Build history of the part. All positions in model axes, mm. A direction names the side the tool comes from. Give positions to 0.01 mm unless a question says otherwise; leave off trailing zeros. Order: outer loops, then holes, each group sorted by start corner. A loop starts at its lowest first (then second) coordinate and runs counter-clockwise, first axis right, second up. Notation, with made-up numbers: (14.25, -6) -> (57.25, -6) arc R15 ccw to (57.25, 19) -> close; hole circle Ø10 at (27, 32). An arc over 180 degrees is marked (long way). One line per question, with ' | ' between items. Start each with the question number.
(1) Which spindle directions (+Z, -Z, +X, -X, +Y, -Y) get a long thin tool onto all of the face, cutting with end or side? Do faces 1 (the face through (10, -30, 23)), 2 (the face through (-23, -33, 41)), 3 (the face through (-14, -35, 50)), 4 (the face through (-25.1, -30.14, 22.86)), 5 (the face through (25.86, -30.14, 26.1)). Say none if no direction does.
(2) Cut at A-A (z = 66). Give the cut face in (x, y).
(3) Pin check, flat tips, straight feed: pin 1 Ø1.5 at (y, z) = (-38, 41.5) entering from -X; pin 2 Ø24 at (x, z) = (-41, 51.5) entering from -Y; pin 3 Ø2.5 at (x, z) = (-23, 74) entering from +Y; pin 4 Ø10.5 at (x, y) = (-37, -24) entering from -Z. Stop position of each tip, or through.
(4) Pull direction Y, two halves, no side cores. Call faces 6 (the face through (15, -30, 77)), 7 (the face through (-21, -34, 50)), 8 (the face through (15, -40, 74)): +Y half, -Y half, draft (parallel to the pull), parting line (faces both ways), or undercut.
(5) Cut at D-D (x = -48.5). Give the cut face in (y, z).
(6) Drill centre lines: L1, parallel to X at y = -26.5, z = 74; L2, parallel to X at y = -30.25, z = 28; L3, parallel to Y at x = -18, z = 64.5. Where is each one in solid material? Low to high. Write a range as from..to.
(7) Cut at B-B (y = -38). Give the cut face in (x, z).
(8) Cut at C-C (y = -26.5). Give the number of separate pieces and of enclosed holes in the cut face, then the cut area to 3 significant figures.
from build123d import *

# Parameters (mm, degrees)
EXTRUDE_1_DEPTH             = 10
EXTRUDE_2_REACH             = 34.619
SKETCH_2_R                  = 10
EXTRUDE_2_DIRECTION_2_DEPTH = 2
SKETCH_6_R                  = 1.65
SKETCH_6_W                  = 14.704506527
SKETCH_6_H                  = 8.520368268
CUT_EXTRUDE_2_DEPTH         = 43.983979574
FILLET_1_R                  = 1
FILLET_2_R                  = 0.5
EXTRUDE_3_DEPTH             = 8
EXTRUDE_4_DEPTH             = 55
SKETCH_9_W                  = 73
SKETCH_9_H                  = 45
CUT_EXTRUDE_3_DEPTH         = 13
SKETCH_10_W                 = 15
SKETCH_10_H                 = 20
CUT_EXTRUDE_4_DEPTH         = 13
SKETCH_11_W                 = 73
SKETCH_11_H                 = 45
CUT_EXTRUDE_6_DEPTH         = 13
SKETCH_12_W                 = 15
SKETCH_12_H                 = 45
SKETCH_12_W_2               = 10
EXTRUDE_5_DEPTH             = 5
FILLET_3_R                  = 3
SKETCH_14_R                 = 1.55
CUT_EXTRUDE_7_DEPTH         = 102.004950374
SKETCH_15_W                 = 8
SKETCH_15_H                 = 22
CUT_EXTRUDE_8_DEPTH         = 20
SKETCH_18_W                 = 5
SKETCH_18_H                 = 45
SKETCH_18_W_2               = 30.3
EXTRUDE_6_DEPTH             = 13
SKETCH_20_R                 = 1.5
CUT_EXTRUDE_9_DEPTH         = 13


with BuildPart() as part:
    # 草图1 → 凸台-拉伸1 (new, symmetric)
    with BuildSketch(Plane.XY):
        with BuildLine():
            Line((-1.15, 3.987480407), (-1.15, 12))
            Line((-1.15, 12), (-4.15, 12))
            Line((-4.15, 12), (-4.15, 4.333301282))
            ThreePointArc((-4.15, 4.333301282), (-4.784308974, 3.620826928), (-5.297685557, 2.816829377))
            Line((-5.297685557, 2.816829377), (-8, -2.265484914))
            Line((-8, -2.265484914), (-8, -30))
            Line((-8, -30), (0, -30))
            Line((0, -30), (0, -8.485281374))
            Line((0, -8.485281374), (4.242640687, -4.242640687))
            ThreePointArc((4.242640687, -4.242640687), (5.999649956, 0.064810571), (4.15, 4.333301282))
            Line((4.15, 4.333301282), (4.15, 12))
            Line((4.15, 12), (1.15, 12))
            Line((1.15, 12), (1.15, 3.987480407))
            ThreePointArc((1.15, 3.987480407), (0, -4.15), (-1.15, 3.987480407))
        make_face()
    extrude(amount=EXTRUDE_1_DEPTH, both=True)

    # 凸台-拉伸2: up to this face of the body (flat: up to its plane)
    extrude_2_end = Plane(part.part.faces().sort_by_distance((-8, -16.132742457, 0))[0])
    # 草图2 → 凸台-拉伸2 (add, up to the picked face)
    with BuildSketch(Plane(origin=(0, 0, 0), x_dir=(0, 0, -1), z_dir=(1, 0, 0)), mode=Mode.PRIVATE) as extrude_2_sk1:
        with Locations((0, -30)):
            Circle(SKETCH_2_R)
    extrude_2_tool1 = split(extrude(extrude_2_sk1.sketch, amount=-EXTRUDE_2_REACH, mode=Mode.PRIVATE), bisect_by=extrude_2_end, keep=Keep.BOTH, mode=Mode.PRIVATE)
    add(extrude_2_tool1.solids().sort_by(Axis((0, -30, 0), (-1, 0, 0)))[0])

    # 草图2 → 凸台-拉伸2 direction 2 (add)
    with BuildSketch(Plane(origin=(0, 0, 0), x_dir=(0, 0, -1), z_dir=(1, 0, 0))):
        with Locations((0, -30)):
            Circle(SKETCH_2_R)
    extrude(amount=EXTRUDE_2_DIRECTION_2_DEPTH)

    # 草图6 → 切除-拉伸2 (cut, through all)
    with BuildSketch(Plane(origin=(4.15, 0, 0), x_dir=(0, 0, -1), z_dir=(1, 0, 0))):
        with Locations(Location((0, 9.5, 0), (0, 0, 90))):
            Circle(SKETCH_6_R)
        with Locations((-12.852253263, 11.760184134)):
            Rectangle(SKETCH_6_W, SKETCH_6_H)
        with Locations((12.852253263, 11.760184134)):
            Rectangle(SKETCH_6_W, SKETCH_6_H)
    extrude(amount=-CUT_EXTRUDE_2_DEPTH, mode=Mode.SUBTRACT)

    # 圆角1
    fillet_1_edges = [part.edges().sort_by_distance(p)[0] for p in [
        (2.65, 7.5, -10),
        (-2.65, 7.5, -10),
        (2.65, 7.5, 10),
        (-2.65, 7.5, 10),
        (2.65, 12, 5.5),
        (-2.65, 12, 5.5),
        (2.65, 12, -5.5),
        (-2.65, 12, -5.5),
    ]]
    fillet(fillet_1_edges, radius=FILLET_1_R)

    # 圆角2
    fillet_2_edges = [part.edges().sort_by_distance(p)[0] for p in [
        (-2.65, 7.5, 5.5),
        (2.65, 7.5, 5.5),
        (2.65, 7.5, -5.5),
        (-2.65, 7.5, -5.5),
    ]]
    fillet(fillet_2_edges, radius=FILLET_2_R)

    # 草图7 → 凸台-拉伸3 (add)
    with BuildSketch(Plane(origin=(2, 0, 0), x_dir=(0, 0, -1), z_dir=(1, 0, 0))):
        with BuildLine():
            Line((0, -20), (-22, -20))
            Line((-22, -20), (-22, -40))
            Line((-22, -40), (0, -40))
            ThreePointArc((0, -40), (10, -30), (0, -20))
        make_face()
    extrude(amount=EXTRUDE_3_DEPTH)

    # 草图8 → 凸台-拉伸4 (add)
    with BuildSketch(Plane.XY.offset(22)):
        Polygon((10, -20), (-26, -20), (-26, -40), (2, -40), (57, -40), (57, -20), align=None)
    extrude(amount=EXTRUDE_4_DEPTH)

    # 草图9 → 切除-拉伸3 (cut)
    with BuildSketch(Plane(origin=(0, -20, 0), x_dir=(1, 0, 0), z_dir=(0, 1, 0))):
        with Locations((15.5, -49.5)):
            Rectangle(SKETCH_9_W, SKETCH_9_H)
    extrude(amount=-CUT_EXTRUDE_3_DEPTH, mode=Mode.SUBTRACT)

    # 草图10 → 切除-拉伸4 (cut)
    with BuildSketch(Plane(origin=(0, 0, 22), x_dir=(-1, 0, 0), z_dir=(0, 0, -1))):
        with Locations((-17.5, -30)):
            Rectangle(SKETCH_10_W, SKETCH_10_H)
    extrude(amount=-CUT_EXTRUDE_4_DEPTH, mode=Mode.SUBTRACT)

    # 草图11 → 切除-拉伸6 (cut)
    with BuildSketch(Plane(origin=(0, -33, 0), x_dir=(1, 0, 0), z_dir=(0, 1, 0))):
        with Locations((15.5, -49.5)):
            Rectangle(SKETCH_11_W, SKETCH_11_H)
    extrude(amount=-CUT_EXTRUDE_6_DEPTH, mode=Mode.SUBTRACT)

    # 草图12 → 凸台-拉伸5 (add)
    with BuildSketch(Plane.XZ.offset(40)):
        with Locations((-13.5, 49.5)):
            Rectangle(SKETCH_12_W, SKETCH_12_H)
        with Locations((47, 49.5)):
            Rectangle(SKETCH_12_W_2, SKETCH_12_H)
    extrude(amount=-EXTRUDE_5_DEPTH)

    # 圆角3
    fillet_3_edges = [part.edges().sort_by_distance(p)[0] for p in [
        (-26, -30, 22),
        (57, -30, 22),
        (-26, -30, 77),
        (57, -30, 77),
        (10, -30, 27),
        (25, -30, 27),
    ]]
    fillet(fillet_3_edges, radius=FILLET_3_R)

    # 草图14 → 切除-拉伸7 (cut, through all)
    with BuildSketch(Plane(origin=(0, -20, 0), x_dir=(1, 0, 0), z_dir=(0, 1, 0))):
        with Locations(Location((-23, -25, 0), (0, 0, 270))):
            Circle(SKETCH_14_R)
        with Locations(Location((54, -25, 0), (0, 0, 270))):
            Circle(SKETCH_14_R)
        with Locations(Location((-23, -74, 0), (0, 0, 270))):
            Circle(SKETCH_14_R)
        with Locations(Location((54, -74, 0), (0, 0, 270))):
            Circle(SKETCH_14_R)
    extrude(amount=-CUT_EXTRUDE_7_DEPTH, mode=Mode.SUBTRACT)

    # 草图15 → 切除-拉伸8 (cut)
    with BuildSketch(Plane(origin=(0, -20, 0), x_dir=(1, 0, 0), z_dir=(0, 1, 0))):
        with Locations((6, -11)):
            Rectangle(SKETCH_15_W, SKETCH_15_H)
    extrude(amount=-CUT_EXTRUDE_8_DEPTH, mode=Mode.SUBTRACT)


with BuildPart() as body_2:
    # of the pieces the cut leaves, the one that is kept (cut_extrude_8_keep)
    add(part.part.solids().sort_by_distance((-26, -20, 25))[0])

    # 草图18 → 凸台-拉伸6 (add)
    with BuildSketch(Plane(origin=(0, -20, 0), x_dir=(1, 0, 0), z_dir=(0, 1, 0))):
        with Locations((-18.5, -49.5)):
            Rectangle(SKETCH_18_W, SKETCH_18_H)
        with Locations((-41.15, -49.5)):
            Rectangle(SKETCH_18_W_2, SKETCH_18_H)
    extrude(amount=-EXTRUDE_6_DEPTH)

    # 草图20 → 切除-拉伸9 (cut)
    with BuildSketch(Plane(origin=(0, -20, 0), x_dir=(1, 0, 0), z_dir=(0, 1, 0))):
        with Locations(Location((-22.89532608, -62.69503523, 0), (0, 0, 270))):
            Circle(SKETCH_20_R)
        with Locations(Location((-51.895321909, -41.179481559, 0), (0, 0, 270))):
            Circle(SKETCH_20_R)
        with Locations((-21.949220364, 0)):
            Circle(SKETCH_20_R)
        with Locations(Location((-51.895321909, -62.69503523, 0), (0, 0, 270))):
            Circle(SKETCH_20_R)
        with Locations(Location((-22.89532608, -41.19503523, 0), (0, 0, 270))):
            Circle(SKETCH_20_R)
    extrude(amount=-CUT_EXTRUDE_9_DEPTH, mode=Mode.SUBTRACT)


solid = body_2.part
Result set:
1) face 1: -Z, +Y, -Y | face 2: +Y | face 3: none | face 4: -Z, -X, +Y, -Y | face 5: +Y, -Y
2) outline: (-56.3, -33) -> (-26, -33) -> (-26, -40) -> (-6, -40) -> (-6, -35) -> (-21, -35) -> (-21, -33) -> (-16, -33) -> (-16, -20) -> (-56.3, -20) -> close; (42, -40) -> (57, -40) -> (57, -20) -> (52, -20) -> (52, -35) -> (42, -35) -> close
3) pin 1: stops at x = -26 | pin 2: stops at y = -33 | pin 3: passes through | pin 4: stops at z = 27
4) face 6: draft | face 7: undercut | face 8: -Y half
5) outline: (-33, 27) -> (-20, 27) -> (-20, 72) -> (-33, 72) -> close
6) L1: x = -26..-24.55, -21.45..52.45, 55.55..57 | L2: x = -56.3..-16, 52..57 | L3: y = -40..-35, -33..-20
7) outline: (-26, 25) arc R3 ccw to (-23, 22) -> (10, 22) -> (10, 24) arc R3 ccw to (7, 27) -> (-6, 27) -> (-6, 72) -> (42, 72) -> (42, 27) -> (28, 27) arc R3 ccw to (25, 24) -> (25, 22) -> (54, 22) arc R3 ccw to (57, 25) -> (57, 74) arc R3 ccw to (54, 77) -> (-23, 77) arc R3 ccw to (-26, 74) -> close; hole circle Ø3.1 at (-23, 25); hole circle Ø3.1 at (-23, 74); hole circle Ø3.1 at (54, 25); hole circle Ø3.1 at (54, 74)
8) separate pieces: 1 | enclosed holes: 8 | area: 2,720 mm2
